Check sheet for the modelled part. Datum: model origin and axes. Units: mm. A direction names the side the tool comes from. Give positions to 0.01 mm unless a question says otherwise; leave off trailing zeros. Loops run counter-clockwise (first coordinate to the right, second up) from the corner with the lowest first, then second, coordinate; pieces in that order, holes last. Notation, with made-up numbers: (-34.75, -37.5) - (-8.75, -37.5) arc R35 cw to (-8.75, -1.5) - close; hole circle Ø3 at (42, 43). An arc over 180 degrees is marked (long way). Answer in a Markdown table with one row per item. Add a question column.
(1) Set-up check for faces 1 (the face through (4.3, -0.1, 2)), 2 (the face through (-2.696, 2.684, 1.972)), 3 (the face through (-2.757, -5, 2)), 4 (the face through (2.757, -5, 2)): record each of +Z, -Z, +X, -X, +Y, -Y from which the full face is reachable in a straight line by a thin tool's end or side.
(2) Sectioned sample at A-A on y = 0. Enter the section's corners in (x, z).
(3) Sectioned sample at D-D on x = 0. Enter the section's corners in (y, z), then the cut area to 3 significant figures.
(4) Draft check along Y on faces 5 (the face through (2.703, 2.698, 1.972)), 6 (the face through (0, -4, 0)), 7 (the face through (0.1, -3.3, 2)). Enter one of: released by +Y, released by -Y, zero draft, split by the parting line, or undercut.
(5) Sectioned sample at B-B on z = 2.45. Enter the section's corners in (x, y), then the cut area to 3 significant figures.
(6) Sectioned sample at C-C on y = 1.5. Enter the section's corners in (x, z), then the cut area to 3 significant figures.
(7) Thickness scan on L1, parallel to X at y = 0, z = 2.85; L2, parallel to X at y = -4, z = 3.15; L3, parallel to X at y = -1.75, z = 1.1. Record the ranges inside material, lowest first.
(8) Go/stop test with flat-tipped pins: P1, Ø0.9, axis at y = -5.5, z = 1, coming from the -X side; P2, Ø1.5, axis at y = -3.5, z = 1, coming from the -X side. Record where each tip stops, or that it passes through.
from build123d import *

# Parameters (mm, degrees)
F1_DEPTH = 4


with BuildPart() as f1:
    # F0 (on Top) → F1 (new body)
    with BuildSketch(Plane.XY):
        with BuildLine():
            ThreePointArc((2.426764, 2.23625), (0, -3.3), (-2.426764, 2.23625))
            ThreePointArc((-2.426764, 2.23625), (-2.699268, 2.69082), (-2.887527, 3.18625))
            ThreePointArc((-2.887527, 3.18625), (-4.299127, -0.08664), (-2.75681, -3.3))
            Line((-2.75681, -3.3), (-2.75681, -6.3))
            Line((-2.75681, -6.3), (2.75681, -6.3))
            Line((2.75681, -6.3), (2.75681, -3.3))
            ThreePointArc((2.75681, -3.3), (4.299127, -0.08664), (2.887527, 3.18625))
            ThreePointArc((2.887527, 3.18625), (2.699268, 2.69082), (2.426764, 2.23625))
        make_face()
    extrude(amount=F1_DEPTH)


solid = f1.part
Reply:
| question | item | result |
|---|---|---|
| 1 | face 1 | +Z, -Z, +X |
| 1 | face 2 | +Z, -Z, +Y |
| 1 | face 3 | +Z, -Z, -X, -Y |
| 1 | face 4 | +Z, -Z, +X, -Y |
| 2 | outline | (-4.3, 0) - (-3.3, 0) - (-3.3, 4) - (-4.3, 4) - close; (3.3, 0) - (4.3, 0) - (4.3, 4) - (3.3, 4) - close |
| 3 | outline | (-6.3, 0) - (-3.3, 0) - (-3.3, 4) - (-6.3, 4) - close |
| 3 | area | 12.0 mm^2 |
| 4 | face 5 | released by +Y |
| 4 | face 6 | zero draft |
| 4 | face 7 | undercut |
| 5 | outline | (-2.89, 3.19) arc R4.3 ccw to (-2.76, -3.3) - (-2.76, -6.3) - (2.76, -6.3) - (2.76, -3.3) arc R4.3 ccw to (2.89, 3.19) arc R3 cw to (2.43, 2.24) arc R3.3 cw (long way) to (-2.43, 2.24) arc R3 cw to start |
| 5 | area | 30.7 mm^2 |
| 6 | outline | (-4.03, 0) - (-2.94, 0) - (-2.94, 4) - (-4.03, 4) - close; (2.94, 0) - (4.03, 0) - (4.03, 4) - (2.94, 4) - close |
| 6 | area | 8.72 mm^2 |
| 7 | L1 | -4.3 to -3.3, 3.3 to 4.3 |
| 7 | L2 | -2.76 to 2.76 |
| 7 | L3 | -3.93 to -2.8, 2.8 to 3.93 |
| 8 | P1 | x = -2.76 |
| 8 | P2 | x = -3.31 |
